Could you check a few things on this model? Use its own coordinates, in mm. Face numbers are marked on the shaded views. A direction names the side the tool comes from. Give positions to 0.01 mm unless a question says otherwise; leave off trailing zeros. Order: outer loops, then holes, each group sorted by start corner. A loop starts at its lowest first (then second) coordinate and runs counter-clockwise, first axis right, second up. Notation, with made-up numbers: (-40, 58.25) -> (-32, 58.25) arc R23 cw to (-32, 83.25) -> close; hole circle Ø8 at (15, 53.5). An arc over 180 degrees is marked (long way). Answer as CSV lines item,"result". Start each with the question number.
(1) We'd pull the mould along X, two halves only. Please class the marked faces 6, 7, 8 and 9: released by +X, released by -X, zero draft, split by the parting line, or undercut.
(2) I want a section at C-C (y = -53.5). Please give me the cut outline in (x, z) (3 decimals), plus the area to 3 significant figures.
(3) On a 3-axis mill with a long thin cutter (end or side, diameter ignored), from which of +Z, -Z, +X, -X, +Y, -Y can I reach the whole of each face in a straight line? I mean the marked faces 1, 2, 3, 4 and 5. Say none if no direction works.
(4) I need wall thicknesses on L1, parallel to Z at x = -33, y = -57.5 (3 decimals); L2, parallel to X at y = -8, z = 18 (3 decimals); L3, parallel to X at y = 7.5, z = -3 (3 decimals). Which ranges of each line are inside material? Lowest first, please.
(5) I want a section at A-A (z = -2). Please give me the cut outline in (x, y) (3 decimals), plus the area to 3 significant figures.
(6) Will these pins go through, and if not, where does the flat tip stop? pin 1 Ø5.5 at (x, y) = (64, -2.5) entering from -Z; pin 2 Ø15 at (x, z) = (44, 28.5) entering from -Y; pin 3 Ø19 at (y, z) = (-20, 21.5) entering from -X (3 decimals); pin 4 Ø3 at (x, z) = (0.5, 45) entering from +Y.
(7) I want a section at B-B (x = 67.5). Please give me the cut outline in (y, z) (3 decimals).
```python
from build123d import *

# Parameters (mm, degrees)
F1_DEPTH  = 63.5
F2_DEPTH  = 25.4
F3_DEPTH  = 7.9375
F2_FACE_W = 50.8
F2_FACE_H = 19.05
F4_DEPTH  = 12.7
F6_R      = 6.35


with BuildPart() as f1:
    # F0 (on Front) → F1 (new body, symmetric)
    with BuildSketch(Plane.XZ):
        Polygon((41.275, -9.525), (41.275, 9.525), (22.225, 9.525), (-41.275, 9.525), (-41.275, -9.525), align=None)
    extrude(amount=F1_DEPTH, both=True)

    # F0 (on Front) → F2 (join, symmetric)
    with BuildSketch(Plane.XZ):
        with BuildLine():
            Line((22.225, 9.525), (41.275, 9.525))
            Line((41.275, 9.525), (41.275, 27.915647))
            ThreePointArc((41.275, 27.915647), (45.211633, 38.379443), (55.069144, 43.653679))
            Line((55.069144, 43.653679), (60.325, 43.653679))
            Line((60.325, 43.653679), (60.325, 62.703679))
            Line((60.325, 62.703679), (54.059947, 62.703679))
            add(Edge.make_bspline(
                [(50.568891, 62.214986), (51.7192, 62.392836), (52.882727, 62.555887), (54.059947, 62.703679)],
                knots=[106.101689, 106.101689, 106.101689, 106.101689, 109.163749, 109.163749, 109.163749, 109.163749], degree=3))
            ThreePointArc((50.568891, 62.214986), (30.227882, 50.163236), (22.225, 27.915647))
            Line((22.225, 27.915647), (22.225, 9.525))
        make_face()
    extrude(amount=F2_DEPTH, both=True)

    # F0 (on Front) → F3 (join, symmetric)
    with BuildSketch(Plane.XZ):
        with BuildLine():
            Line((-41.275, 9.525), (22.225, 9.525))
            Line((22.225, 9.525), (22.225, 27.915647))
            ThreePointArc((22.225, 27.915647), (30.227882, 50.163236), (50.568891, 62.214986))
            add(Edge.make_bspline(
                [(-41.275, 9.525), (-13.280101, 32.121023), (10.710167, 56.052397), (50.568891, 62.214986)],
                knots=[0, 0, 0, 0, 106.101689, 106.101689, 106.101689, 106.101689], degree=3))
        make_face()
    extrude(amount=F3_DEPTH, both=True)

    # F2_face (on face) → F4 (join)
    with BuildSketch(Plane(origin=(60.325, 0, 53.178679), x_dir=(0, 1, 0), z_dir=(1, 0, 0))):
        Rectangle(F2_FACE_W, F2_FACE_H)
    extrude(amount=F4_DEPTH)

    # F0 (on Front) → F5 (revolve)
    with BuildSketch(Plane.XZ):
        Polygon((83.573606, 62.703679), (83.573606, 43.653679), (83.573606, 38.1), (111.125, 38.1), (111.125, 66.675), (83.573606, 66.675), align=None)
    revolve(axis=Axis((83.573606, 0, 40.87684), (0, 0, -1)))

    # F6
    f6_edges = [f1.edges().sort_by_distance(p)[0] for p in [
        (-41.275, -63.5, 0),
        (41.275, -63.5, 0),
        (41.275, 63.5, 0),
        (-41.275, 63.5, 0),
    ]]
    fillet(f6_edges, radius=F6_R)


solid = f1.part
```
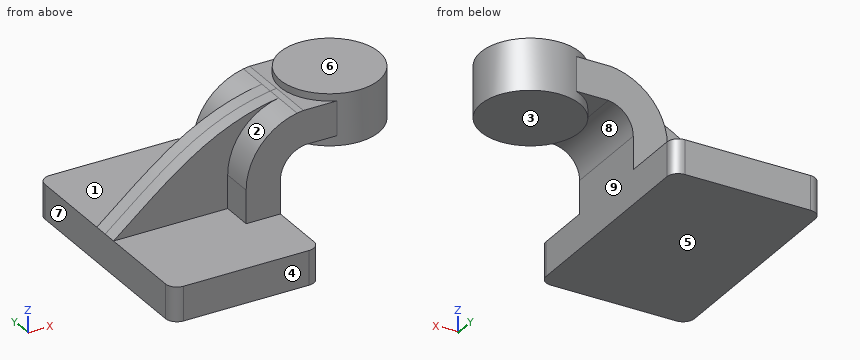
Final values:
1,face 6,"zero draft"
1,face 7,"released by -X"
1,face 8,"undercut"
1,face 9,"released by +X"
2,outline,"(-41.275, -9.525) -> (41.275, -9.525) -> (41.275, 9.525) -> (-41.275, 9.525) -> close"
2,area,"1,570 mm²"
3,face 1,"+Z, -X, +Y"
3,face 2,"+Z, -X, -Y"
3,face 3,"-Z, +X, +Y, -Y"
3,face 4,"+Z, -Z, +X, -X, -Y"
3,face 5,"-Z, +X, -X, +Y, -Y"
4,L1,"-9.525 to 9.525"
4,L2,"22.225 to 41.275"
4,L3,"-41.275 to 41.275"
5,outline,"(-41.275, -57.15) arc R6.35 ccw to (-34.925, -63.5) -> (34.925, -63.5) arc R6.35 ccw to (41.275, -57.15) -> (41.275, 57.15) arc R6.35 ccw to (34.925, 63.5) -> (-34.925, 63.5) arc R6.35 ccw to (-41.275, 57.15) -> close"
5,area,"10,400 mm²"
6,pin 1,"z = 38.1"
6,pin 2,"y = -25.4"
6,pin 3,"x = 22.225"
6,pin 4,"through"
7,outline,"(-25.4, 43.654) -> (-22.377, 43.654) -> (-22.377, 38.1) -> (22.377, 38.1) -> (22.377, 43.654) -> (25.4, 43.654) -> (25.4, 62.704) -> (22.377, 62.704) -> (22.377, 66.675) -> (-22.377, 66.675) -> (-22.377, 62.704) -> (-25.4, 62.704) -> close"
